```python
from build123d import *

# Parameters (mm, degrees)
BOSS_EXTRUDE1_DEPTH      = 28
CUT_EXTRUDE1_DEPTH       = 11
CUT_EXTRUDE2_REACH       = 30
SKETCH3_R                = 1.35
FILLET1_R                = 3.98
SKETCH4_R                = 5
BOSS_EXTRUDE2_DEPTH      = 7
SKETCH6_W                = 1.4
SKETCH6_H                = 3.75
CUT_EXTRUDE3_DEPTH       = 17.351430022
SKETCH5_R                = 2.5
BOSS_EXTRUDE3_DEPTH      = 7
BOSS_EXTRUDE3_DEPTH_BACK = 7
SKETCH7_W                = 15.4
SKETCH7_H                = 14
CUT_EXTRUDE4_DEPTH       = 0.2
CUT_EXTRUDE5_DEPTH       = 12


with BuildPart() as part:
    # Sketch1 → Boss-Extrude1 (new body)
    with BuildSketch(Plane.XY):
        Polygon((8, 10), (18, 0), (8, -10), (-8, -10), (-18, 0), (-8, 10), align=None)
    extrude(amount=-BOSS_EXTRUDE1_DEPTH)

    # Sketch2 → Cut-Extrude1 (cut, symmetric)
    with BuildSketch(Plane(origin=(0, 0, 0), x_dir=(1, 0, 0), z_dir=(0, 1, 0))):
        Polygon((-18, 5), (-10.5, 5), (-10.5, 16.8), (-9.4, 22), (-9.4, 28), (-18, 28), align=None)
    cut_extrude1 = extrude(amount=CUT_EXTRUDE1_DEPTH, both=True, mode=Mode.SUBTRACT)

    # Mirror1: Cut-Extrude1 across plane
    add(cut_extrude1.mirror(Plane(origin=(0, 0, 0), x_dir=(0, 0, 1), z_dir=(1, 0, 0))), mode=Mode.SUBTRACT)

    # Sketch3 → Cut-Extrude2 (cut, up to next)
    with BuildSketch(Plane.XY, mode=Mode.PRIVATE) as cut_extrude2_sk1:
        with Locations((-12.5, 0)):
            Circle(SKETCH3_R)
    cut_extrude2_tool1 = extrude(cut_extrude2_sk1.sketch, amount=-CUT_EXTRUDE2_REACH, mode=Mode.PRIVATE) & part.part
    add(cut_extrude2_tool1.solids().sort_by_distance((-12.5, 0, 0))[0], mode=Mode.SUBTRACT)
    # Sketch3 → Cut-Extrude2 (cut, up to next)
    with BuildSketch(Plane.XY, mode=Mode.PRIVATE) as cut_extrude2_sk2:
        with Locations((12.5, 0)):
            Circle(SKETCH3_R)
    cut_extrude2_tool2 = extrude(cut_extrude2_sk2.sketch, amount=-CUT_EXTRUDE2_REACH, mode=Mode.PRIVATE) & part.part
    add(cut_extrude2_tool2.solids().sort_by_distance((12.5, 0, 0))[0], mode=Mode.SUBTRACT)

    # Fillet1
    fillet1_edges = [part.edges().sort_by_distance(p)[0] for p in [
        (-18, 0, -2.5),
        (18, 0, -2.5),
    ]]
    fillet(fillet1_edges, radius=FILLET1_R)

    # Sketch4 → Boss-Extrude2 (add)
    with BuildSketch(Plane(origin=(0, 0, -28), x_dir=(-1, 0, 0), z_dir=(0, 0, -1))):
        Circle(SKETCH4_R)
    extrude(amount=BOSS_EXTRUDE2_DEPTH)

    # Sketch6 → Cut-Extrude3 (cut, symmetric)
    with BuildSketch(Plane(origin=(0, 0, 0), x_dir=(0, 0, -1), z_dir=(1, 0, 0))):
        with Locations((30.1, 3.125)):
            Rectangle(SKETCH6_W, SKETCH6_H)
        with Locations((32.9, 3.125)):
            Rectangle(SKETCH6_W, SKETCH6_H)
    cut_extrude3 = extrude(amount=CUT_EXTRUDE3_DEPTH, both=True, mode=Mode.SUBTRACT)

    # Mirror2: Cut-Extrude3 across plane
    add(cut_extrude3.mirror(Plane.ZX), mode=Mode.SUBTRACT)

    # Sketch5 → Boss-Extrude3 (add, two sides)
    with BuildSketch(Plane(origin=(0, 0, -35), x_dir=(-1, 0, 0), z_dir=(0, 0, -1))) as boss_extrude3_sk:
        Circle(SKETCH5_R)
    extrude(amount=BOSS_EXTRUDE3_DEPTH)
    extrude(boss_extrude3_sk.sketch, amount=-BOSS_EXTRUDE3_DEPTH_BACK)

    # Sketch7 → Cut-Extrude4 (cut)
    with BuildSketch(Plane.XY):
        Rectangle(SKETCH7_W, SKETCH7_H)
    extrude(amount=-CUT_EXTRUDE4_DEPTH, mode=Mode.SUBTRACT)

    # Sketch8 → Cut-Extrude5 (cut)
    with BuildSketch(Plane.XY.offset(-0.2)):
        Polygon((-6, 5), (6, 5), (6, -3.5), (4, -3.5), (4, -5), (2, -5), (2, -6.5), (-2, -6.5), (-2, -5), (-4, -5), (-4, -3.5), (-6, -3.5), align=None)
    extrude(amount=-CUT_EXTRUDE5_DEPTH, mode=Mode.SUBTRACT)


solid = part.part
```
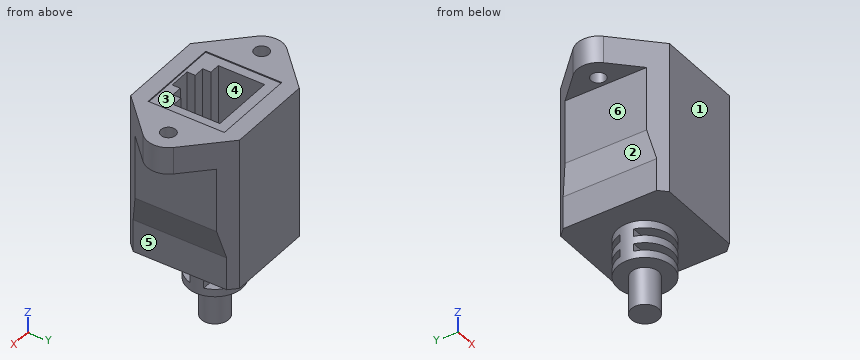
Check sheet for the modelled part. Datum: model origin and axes. Units: mm. Face numbers are marked on the shaded views. A direction names the side the tool comes from. Round coordinates to 2 decimals unless told otherwise and drop trailing zeros. Order: outer loops, then holes, each group sorted by start corner. A loop starts at its lowest first (then second) coordinate and runs counter-clockwise, first axis right, second up. Notation, with made-up numbers: M 26,-6.5 L 30,-6.5 A19 ccw 30,25.5 Z; hole C 7,52.5 d11. An arc over 180 degrees is marked long. Answer in a Markdown table with one row per item.
(1) Section check B-B on z = -27.5. Record the boundary of the cut face in (x, y), plus the area to 3 significant figures.
Findings:
| item | result |
|---|---|
| outline | M -9.4,-8.6 L -8,-10 L 8,-10 L 9.4,-8.6 L 9.4,8.6 L 8,10 L -8,10 L -9.4,8.6 Z |
| area | 372 mm^2 |
(2) Set-up check for the marked faces 4, 5 and 6: record each of +Z, -Z, +X, -X, +Y, -Y from which the full face is reachable in a straight line by a thin tool's end or side.
Findings:
| item | result |
|---|---|
| face 4 | +Z |
| face 5 | -Z, +X, +Y, -Y |
| face 6 | -Z, -X, +Y, -Y |
(3) Gauge pin test, flat ends, axial feed: pin 1 (4 mm diameter, centred on x = 11, y = -6.5, fed in from -Z); pin 2 (1.5 mm diameter, centred on x = 3.5, z = -33, fed in from -Y); pin 3 (8 mm diameter, centred on x = 11, y = 4, fed in from +Z); pin 4 (1.6 mm diameter, centred on y = -5.5, z = -6, fed in from +X). Record the tip position at first contact, or that the pin passes through.
Findings:
| item | result |
|---|---|
| pin 1 | stops at z = -28 |
| pin 2 | stops at y = -3.96 |
| pin 3 | stops at z = 0 |
| pin 4 | stops at x = 10.5 |
(4) Material ranges on line 1 along Y through (x, z) = (12, -1); line 2 along X through (y, z) = (2.5, -5.5); line 3 along Z through (x, y) = (6.5, 0.5), recorded low to high. Write a range as from..to.
Findings:
| item | result |
|---|---|
| line 1 | y = -6..-1.25, 1.25..6 |
| line 2 | x = -10.5..-6, 6..10.5 |
| line 3 | z = -28..-0.2 |
(5) Draft check along X on the marked faces 1, 2 and 3. Enter one of: +X half, -X half, draft (parallel to the pull), parting line (faces both ways), or undercut.
Findings:
| item | result |
|---|---|
| face 1 | draft |
| face 2 | -X half |
| face 3 | undercut |
(6) Section check C-C on y = 0. Give the number of separate pieces and of enclosed holes in the cut face, plus the area to 3 significant figures.
Findings:
| item | result |
|---|---|
| separate pieces | 3 |
| enclosed holes | 0 |
| area | 559 mm^2 |
(7) Section check D-D on x = -7. Record the boundary of the cut face in (y, z).
Findings:
| item | result |
|---|---|
| outline | M -10,-28 L 10,-28 L 10,0 L 7,0 L 7,-0.2 L -7,-0.2 L -7,0 L -10,0 Z |
(8) Section check A-A on x = 12.5. Record the boundary of the cut face in (y, z).
Findings:
| item | result |
|---|---|
| outline | M -5.5,-5 L -1.35,-5 L -1.35,0 L -5.5,0 Z; M 1.35,-5 L 5.5,-5 L 5.5,0 L 1.35,0 Z |
